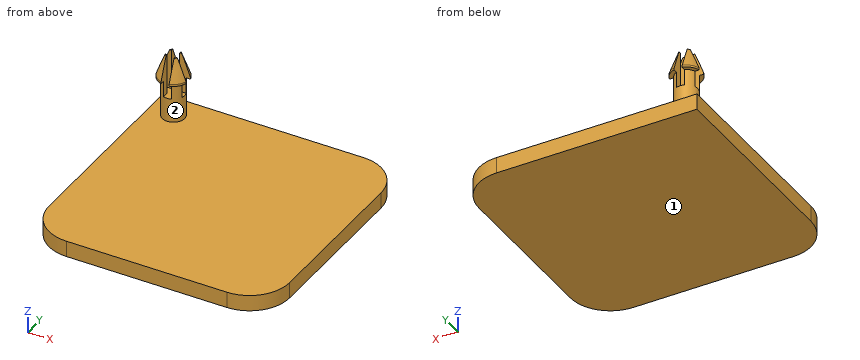
```python
from build123d import *

# Parameters (mm, degrees)
F0_W       = 30
F0_H       = 30
F1_DEPTH   = 2
F2_R       = 5
F3_R       = 1.4
F4_DEPTH   = 5
F5_R       = 1.9
F6_DEPTH   = 3
F7_W       = 1
F7_H       = 1.4164627314
F7_H_2     = 0.9670745373
F8_DEPTH   = 5
F9_SIZE2   = 1
F9_SIZE    = 2.7474774195
F9_2_SIZE2 = 1
F9_2_SIZE  = 2.7474774195
F9_3_SIZE2 = 1
F9_3_SIZE  = 2.7474774195
F9_4_SIZE2 = 1
F9_4_SIZE  = 2.7474774195


with BuildPart() as f1:
    # F0 (on Top) → F1 (new body)
    with BuildSketch(Plane.XY):
        Rectangle(F0_W, F0_H)
    extrude(amount=F1_DEPTH)

    # F2
    f2_edges = [f1.edges().sort_by_distance(p)[0] for p in [
        (-15, -15, 1),
        (15, -15, 1),
        (15, 15, 1),
    ]]
    fillet(f2_edges, radius=F2_R)

    # F3 (on face) → F4 (join)
    with BuildSketch(Plane.XY.offset(2)):
        with Locations((-12, 12)):
            Circle(F3_R)
    extrude(amount=F4_DEPTH)

    # F5 (on face) → F6 (join)
    with BuildSketch(Plane.XY.offset(7)):
        with Locations((-12, 12)):
            Circle(F5_R)
    extrude(amount=F6_DEPTH)

    # F7 (on face) → F8 (cut)
    with BuildSketch(Plane.XY.offset(10)):
        Polygon((-11.5, 11.5164627314), (-9.9080650799, 11.5164627314), (-10.1625583792, 12.4835372686), (-11.5, 12.4835372686), align=None)
        with Locations((-12, 10.8082313657)):
            Rectangle(F7_W, F7_H)
        with Locations((-12, 12)):
            Rectangle(F7_W, F7_H_2)
        Polygon((-13.8374416208, 11.5164627314), (-12.5, 11.5164627314), (-12.5, 12.4835372686), (-14.0919349201, 12.4835372686), align=None)
        with Locations((-12, 13.1917686343)):
            Rectangle(F7_W, F7_H)
    extrude(amount=-F8_DEPTH, mode=Mode.SUBTRACT)

    # F9
    f9_edges = [f1.edges().sort_by_distance(p)[0] for p in [
        (-10.650485, 13.337464, 10),
    ]]
    f9_side = f1.faces().sort_by_distance((-10.650485, 13.337464, 8.5))[0]
    chamfer(f9_edges, length=F9_SIZE, length2=F9_SIZE2, reference=f9_side)

    # F9#2
    f9_2_edges = [f1.edges().sort_by_distance(p)[0] for p in [
        (-10.650485, 10.662536, 10),
    ]]
    f9_2_side = f1.faces().sort_by_distance((-10.650485, 10.662536, 8.5))[0]
    chamfer(f9_2_edges, length=F9_2_SIZE, length2=F9_2_SIZE2, reference=f9_2_side)

    # F9#3
    f9_3_edges = [f1.edges().sort_by_distance(p)[0] for p in [
        (-13.349515, 13.337464, 10),
    ]]
    f9_3_side = f1.faces().sort_by_distance((-13.349515, 13.337464, 8.5))[0]
    chamfer(f9_3_edges, length=F9_3_SIZE, length2=F9_3_SIZE2, reference=f9_3_side)

    # F9#4
    f9_4_edges = [f1.edges().sort_by_distance(p)[0] for p in [
        (-13.349515, 10.662536, 10),
    ]]
    f9_4_side = f1.faces().sort_by_distance((-13.349515, 10.662536, 8.5))[0]
    chamfer(f9_4_edges, length=F9_4_SIZE, length2=F9_4_SIZE2, reference=f9_4_side)


solid = f1.part
```
Check sheet for the modelled part. Datum: model origin and axes. Units: mm. Face numbers are marked on the shaded views. Round coordinates to 2 decimals unless told otherwise and drop trailing zeros. Order: outer loops, then holes, each group sorted by start corner. A loop starts at its lowest first (then second) coordinate and runs counter-clockwise, first axis right, second up. Notation, with made-up numbers: (81.5, 84) -> (110.5, 84) arc R28 ccw to (110.5, 104) -> close; hole circle Ø6 at (-39.5, 74). An arc over 180 degrees is marked (long way). One line per item, written item: value. Start each with the question number.
Q1. Gauge pin test, flat ends, axial feed: pin 1 Ø1.1 at (x, y) = (-10.5, 10.5) entering from -Z; pin 2 Ø1.5 at (x, z) = (-13.5, 8) entering from +Y; pin 3 Ø0.7 at (y, z) = (10.5, 7) entering from +X; pin 4 Ø1.5 at (x, z) = (-13.5, 7) entering from -Y. Record the tip position at first contact, or that the pin passes through.
Q2. Cross-section at A-A (z = 5.5). Record the boundary of the cut face in (x, y).
Q3. Cross-section at C-C (x = -4.5). Record the boundary of the cut face in (y, z), and give its area (3 significant figures).
Q4. Mould release check, pull along Z, two halves, no side actions. Record for the marked faces 1 and 2: pulls with the +Z half, pulls with the -Z half, needs draft (parallel to the pull), parting line crosses it, or undercut.
Q5. Cross-section at B-B (y = 12). Record the boundary of the cut face in (x, z).
Q6. Thickness scan on line 1 (Z direction, x = 13, y = 2.5); line 2 (Y direction, x = -12.75, z = 3.25); line 3 (Y direction, x = 12.5, z = 1). Record the ranges inside material, lowest first.
Completed:
1. pin 1: stops at z = 0
1. pin 2: stops at y = 13.55
1. pin 3: stops at x = -10.49
1. pin 4: stops at y = 10.25
2. outline: (-13.31, 11.52) arc R1.4 ccw to (-12.5, 10.69) -> (-12.5, 11.52) -> close; (-13.31, 12.48) -> (-12.5, 12.48) -> (-12.5, 13.31) arc R1.4 ccw to start; (-11.5, 10.69) arc R1.4 ccw to (-10.69, 11.52) -> (-11.5, 11.52) -> close; (-11.5, 12.48) -> (-10.69, 12.48) arc R1.4 ccw to (-11.5, 13.31) -> close
3. outline: (-15, 0) -> (15, 0) -> (15, 2) -> (-15, 2) -> close
3. area: 60.0 mm²
4. face 1: pulls with the -Z half
4. face 2: undercut
5. outline: (-15, 0) -> (14.58, 0) -> (14.58, 2) -> (-10.6, 2) -> (-10.6, 5) -> (-13.4, 5) -> (-13.4, 2) -> (-15, 2) -> close
6. line 1: z = 0 to 2
6. line 2: y = 10.82 to 13.18
6. line 3: y = -14.33 to 14.33
